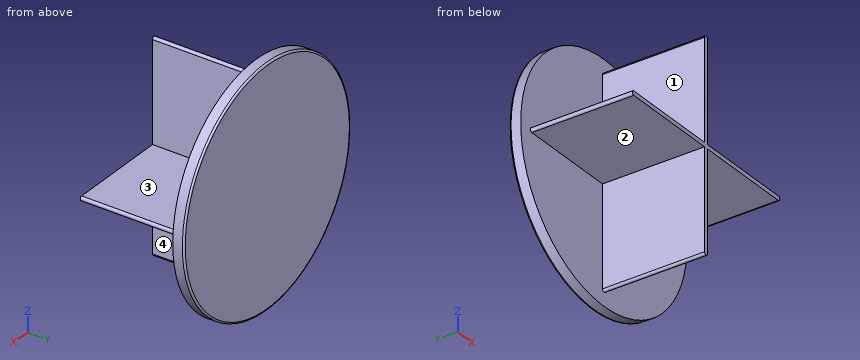
from build123d import *

# Parameters (mm, degrees)
SKETCH1_R           = 527.05
BOSS_EXTRUDE1_DEPTH = 50.8
FILLET1_R           = 7.62
BOSS_EXTRUDE2_DEPTH = 457.2


with BuildPart() as part:
    # Sketch1 → Boss-Extrude1 (new body)
    with BuildSketch(Plane(origin=(0, 0, 0), x_dir=(1, 0, 0), z_dir=(0, 1, 0))):
        with Locations(Location((0, 0, 0), (0, 0, 270))):
            Circle(SKETCH1_R)
    extrude(amount=BOSS_EXTRUDE1_DEPTH)

    # Fillet1
    fillet1_edges = [part.edges().sort_by_distance(p)[0] for p in [
        (0, 50.8, -527.05),
    ]]
    fillet(fillet1_edges, radius=FILLET1_R)

    # Sketch2 → Boss-Extrude2 (add)
    with BuildSketch(Plane.XZ):
        with BuildLine():
            Line((-9.525, 457.2), (-9.525, -457.2))
            ThreePointArc((-9.525, -457.2), (0, -466.725), (9.525, -457.2))
            Line((9.525, -457.2), (9.525, 457.2))
            ThreePointArc((9.525, 457.2), (0, 466.725), (-9.525, 457.2))
        make_face()
        with BuildLine():
            Line((-457.2, -9.525), (457.2, -9.525))
            ThreePointArc((457.2, -9.525), (466.725, 0), (457.2, 9.525))
            Line((457.2, 9.525), (-457.2, 9.525))
            ThreePointArc((-457.2, 9.525), (-466.725, 0), (-457.2, -9.525))
        make_face()
    extrude(amount=BOSS_EXTRUDE2_DEPTH)


solid = part.part
Geometry check sheet. Reference: the model listing, model coordinates, mm. Face numbers are marked on the shaded views. A direction names the side the tool comes from. Round coordinates to 2 decimals unless told otherwise and drop trailing zeros. Loops run counter-clockwise (first coordinate to the right, second up) from the corner with the lowest first, then second, coordinate; pieces in that order, holes last. Notation, with made-up numbers: (88, 22.25) -> (145, 22.25) arc R22 cw to (145, 49.25) -> close; hole circle Ø8 at (84, 20.25). An arc over 180 degrees is marked (long way). Answer as a JSON object with one key per item and string values. Group by question number.
Item 1: Thickness scan on line 1 along Z through (x, y) = (-108, -199.5) (3 decimals); line 2 along Y through (x, z) = (-204, -295). Record the ranges inside material, lowest first.
Item 2: Depth check by flat-ended pin: pin 1 Ø2 at (x, y) = (-375, -199.5) entering from -Z (3 decimals); pin 2 Ø5 at (x, y) = (353.5, -335.5) entering from +Z (3 decimals); pin 3 Ø5 at (x, z) = (195.5, 14.5) entering from -Y. Enter the tip coordinate at first touch or a pass-through.
Item 3: Set-up check for the marked faces 1, 2, 3 and 4: record each of +Z, -Z, +X, -X, +Y, -Y from which the full face is reachable in a straight line by a thin tool's end or side.
Item 4: Cross-section at A-A, the plane y = -152. Record the cut outline in (x, z) (3 decimals), plus the area to 3 significant figures.
Determined:
{
 "1": {"line 1": "z = -9.525 to 9.525", "line 2": "y = 0 to 50.8"},
 "2": {"pin 1": "stops at z = -9.525", "pin 2": "stops at z = 9.525", "pin 3": "stops at y = 0"},
 "3": {"face 1": "+Z, -X, -Y", "face 2": "-Z, -X, -Y", "face 3": "+Z, +X, -Y", "face 4": "-Z, +X, -Y"},
 "4": {"outline": "(-457.2, -9.525) -> (-9.525, -9.525) -> (-9.525, -457.2) arc R9.525 ccw to (9.525, -457.2) -> (9.525, -9.525) -> (457.2, -9.525) arc R9.525 ccw to (457.2, 9.525) -> (9.525, 9.525) -> (9.525, 457.2) arc R9.525 ccw to (-9.525, 457.2) -> (-9.525, 9.525) -> (-457.2, 9.525) arc R9.525 ccw to start", "area": "35,000 mm²"}
}
